Check sheet for the modelled part. Datum: model origin and axes. Units: mm. A direction names the side the tool comes from. Give positions to 0.01 mm unless a question says otherwise; leave off trailing zeros. Order: outer loops, then holes, each group sorted by start corner. A loop starts at its lowest first (then second) coordinate and runs counter-clockwise, first axis right, second up. Notation, with made-up numbers: (-34.5, 68) - (8.5, 68) arc R11 cw to (8.5, 72) - close; hole circle Ø6 at (29, -38.5). An arc over 180 degrees is marked (long way). Answer in a Markdown table with one row per item.
from build123d import *

# Parameters (mm, degrees)
F0_W     = 203.2
F0_H     = 101.6
F0_R     = 7.14375
F1_DEPTH = 12.7
F2_W     = 12.7
F2_H     = 279.4
F3_DEPTH = 152.4
F5_DEPTH = 107.951
F6_SIZE  = 25.4


with BuildPart() as f1:
    # F0 (on Top) → F1 (new body)
    with BuildSketch(Plane.XY):
        Rectangle(F0_W, F0_H)
        with Locations((-76.2, -25.4)):
            Circle(F0_R, mode=Mode.SUBTRACT)
        with Locations((76.2, -25.4)):
            Circle(F0_R, mode=Mode.SUBTRACT)
        with Locations((-76.2, 25.4)):
            Circle(F0_R, mode=Mode.SUBTRACT)
        with Locations((76.2, 25.4)):
            Circle(F0_R, mode=Mode.SUBTRACT)
    extrude(amount=F1_DEPTH)

    # F2 (on face) → F3 (join)
    with BuildSketch(Plane(origin=(0, 0, 0), x_dir=(1, 0, 0), z_dir=(0, 0, -1))):
        with Locations((0, -88.9)):
            Rectangle(F2_W, F2_H)
    extrude(amount=F3_DEPTH)

    # F4 (on face) → F5 (cut, through all)
    with BuildSketch(Plane(origin=(-6.35, 0, 0), x_dir=(0, -1, 0), z_dir=(-1, 0, 0))):
        Polygon((50.8, -25.4), (-76.2, -152.4), (50.8, -152.4), align=None)
    extrude(amount=-F5_DEPTH, mode=Mode.SUBTRACT)

    # F6
    f6_edges = [f1.edges().sort_by_distance(p)[0] for p in [
        (0, 228.6, 0),
    ]]
    chamfer(f6_edges, length=F6_SIZE)


solid = f1.part
(1) Access from +Z, -Z, +X, -X, +Y, -Y to the whole of each face (thin tool, end or side, straight path). Record for faces 4 (the cylindrical face through (83.014, 27.546, 6.261)), 5 (the flat face through (0, 126, 0)), 6 (the flat face through (-6.35, 122, -75)), 7 (the flat face through (53, 1, 0)).
Geometry says:
| item | result |
|---|---|
| face 4 | +Z, -Z |
| face 5 | +Z, +X, -X, +Y |
| face 6 | -Z, -X, +Y, -Y |
| face 7 | -Z, +X, +Y, -Y |
(2) Cross-section at B-B, the plane y = -25.4. Record the cut outline in (x, z).
Geometry says:
| item | result |
|---|---|
| outline | (-101.6, 0) - (-83.34, 0) - (-83.34, 12.7) - (-101.6, 12.7) - close; (-69.06, 0) - (-6.35, 0) - (-6.35, -50.8) - (6.35, -50.8) - (6.35, 0) - (69.06, 0) - (69.06, 12.7) - (-69.06, 12.7) - close; (83.34, 0) - (101.6, 0) - (101.6, 12.7) - (83.34, 12.7) - close |
(3) Mould release check, pull along X, two halves, no side actions. Record for faces 1 (the flat face through (-101.6, -1, 6)), 2 (the flat face through (-1, 1, 12.7)), 3 (the cylindrical face through (83.014, -23.254, 6.261)): pulls with the +X half, pulls with the -X half, needs draft (parallel to the pull), parting line crosses it, or undercut.
Geometry says:
| item | result |
|---|---|
| face 1 | pulls with the -X half |
| face 2 | needs draft |
| face 3 | undercut |
(4) Thickness scan on L1, parallel to X at y = 25, z = 5; L2, parallel to Y at x = -76, z = 10; L3, parallel to X at y = 23, z = 4. Record the ranges inside material, lowest first.
Geometry says:
| item | result |
|---|---|
| L1 | -101.6 to -83.33, -69.07 to 69.07, 83.33 to 101.6 |
| L2 | -50.8 to -32.54, -18.26 to 18.26, 32.54 to 50.8 |
| L3 | -101.6 to -82.93, -69.47 to 69.47, 82.93 to 101.6 |
(5) Cross-section at C-C, the plane y = 25.4. Record the cut outline in (x, z), then the cut area to 3 significant figures.
Geometry says:
| item | result |
|---|---|
| outline | (-101.6, 0) - (-83.34, 0) - (-83.34, 12.7) - (-101.6, 12.7) - close; (-69.06, 0) - (-6.35, 0) - (-6.35, -101.6) - (6.35, -101.6) - (6.35, 0) - (69.06, 0) - (69.06, 12.7) - (-69.06, 12.7) - close; (83.34, 0) - (101.6, 0) - (101.6, 12.7) - (83.34, 12.7) - close |
| area | 3,510 mm² |
(6) Cross-section at A-A, the plane x = -76.2. Record the cut outline in (y, z).
Geometry says:
| item | result |
|---|---|
| outline | (-50.8, 0) - (-32.54, 0) - (-32.54, 12.7) - (-50.8, 12.7) - close; (-18.26, 0) - (18.26, 0) - (18.26, 12.7) - (-18.26, 12.7) - close; (32.54, 0) - (50.8, 0) - (50.8, 12.7) - (32.54, 12.7) - close |
(7) Gauge pin test, flat ends, axial feed: P1, Ø13, axis at x = 76.2, y = -25.4, coming from the +Z side; P2, Ø18.5, axis at x = 76.2, y = 25.4, coming from the -Z side; P3, Ø14, axis at x = -0.5, y = 119, coming from the +Z side; P4, Ø8, axis at y = 86, z = -48, coming from the +X side. Record the tip position at first contact, or that the pin passes through.
Geometry says:
| item | result |
|---|---|
| P1 | through |
| P2 | z = 0 |
| P3 | z = 0 |
| P4 | x = 6.35 |
(8) Cross-section at D-D, the plane z = -115. Record the cut outline in (x, y).
Geometry says:
| item | result |
|---|---|
| outline | (-6.35, 38.8) - (6.35, 38.8) - (6.35, 228.6) - (-6.35, 228.6) - close |
